Check sheet for the modelled part. Datum: model origin and axes. Units: mm. Face numbers are marked on the shaded views. Round coordinates to 2 decimals unless told otherwise and drop trailing zeros. Loops run counter-clockwise (first coordinate to the right, second up) from the corner with the lowest first, then second, coordinate; pieces in that order, holes last. Notation, with made-up numbers: (40.25, 44) -> (77.25, 44) arc R24 cw to (77.25, 72) -> close; hole circle Ø10 at (85.25, 88.5). An arc over 180 degrees is marked (long way). One line per item, written item: value. Start each with the question number.
1. Release check for a two-part mould opening along Z. For the marked faces 1, 2 and 3 record: +Z half, -Z half, draft (parallel to the pull), parting line (faces both ways), or undercut.
2. Cross-section at A-A on z = 0. Record the cut outline in (x, y), then the cut area to 3 significant figures.
3. Cross-section at C-C on x = 3.8. Record the cut outline in (y, z).
4. Cross-section at D-D on z = -3.75. Record the cut outline in (x, y), then the cut area to 3 significant figures.
5. Material ranges on L1, parallel to Y at x = 4.75, z = 0; L2, parallel to X at y = 16.5, z = -2.25; L3, parallel to Y at x = 3.8, z = 1, recorded low to high.
6. Go/stop test with flat-tipped pins: pin 1 (1.5 mm diameter, centred on x = 4, y = -15.5, fed in from +Z); pin 2 (1 mm diameter, centred on y = 7.5, z = -2, fed in from +X); pin 3 (1.5 mm diameter, centred on x = 1, z = 2, fed in from +Y); pin 4 (2 mm diameter, centred on x = 4.5, z = 1.5, fed in from +Y). Record where each tip stops, or that it passes through.
7. Cross-section at B-B on y = 0. Record the cut outline in (x, z).
from build123d import *

# Parameters (mm, degrees)
SKETCH1_R           = 4.318
BOSS_EXTRUDE1_DEPTH = 5.842
BOSS_EXTRUDE2_DEPTH = 2.6162
SKETCH3_R           = 2.7305
CUT_EXTRUDE1_DEPTH  = 3.2258


with BuildPart() as part:
    # Sketch1 → Boss-Extrude1 (new body)
    with BuildSketch(Plane(origin=(0, 0, 0), x_dir=(0, 0, -1), z_dir=(1, 0, 0))):
        Circle(SKETCH1_R)
    extrude(amount=BOSS_EXTRUDE1_DEPTH)

    # Sketch2 → Boss-Extrude2 (add)
    with BuildSketch(Plane.ZY):
        with BuildLine():
            Line((-2.54, 17.140843061), (-4.226068598, 0.886266441))
            ThreePointArc((-4.226068598, 0.886266441), (0, 4.318), (4.226068598, 0.886266441))
            Line((4.226068598, 0.886266441), (2.54, 17.140843061))
            ThreePointArc((2.54, 17.140843061), (0, 19.431), (-2.54, 17.140843061))
        make_face()
    boss_extrude2 = extrude(amount=-BOSS_EXTRUDE2_DEPTH)

    # Mirror1: Boss-Extrude2 across plane
    add(boss_extrude2.mirror(Plane.ZX))

    # Sketch3 → Cut-Extrude1 (cut)
    with BuildSketch(Plane(origin=(5.842, 0, 0), x_dir=(0, 0, -1), z_dir=(1, 0, 0))):
        Circle(SKETCH3_R)
    extrude(amount=-CUT_EXTRUDE1_DEPTH, mode=Mode.SUBTRACT)


solid = part.part
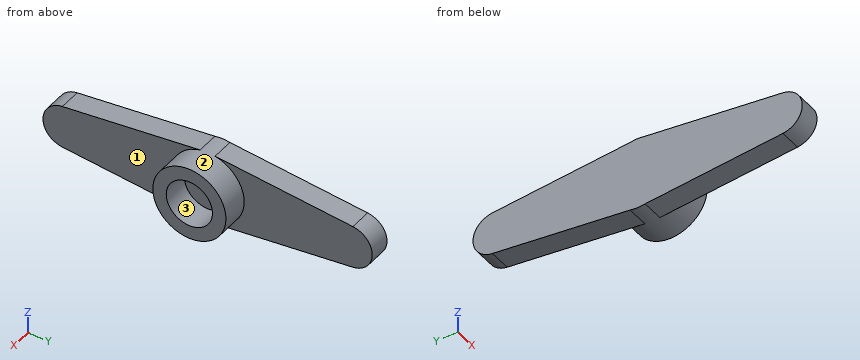
Taken from the geometry:
1. face 1: draft
1. face 2: parting line
1. face 3: undercut
2. outline: (0, -19.43) -> (2.62, -19.43) -> (2.62, -4.32) -> (5.84, -4.32) -> (5.84, -2.73) -> (2.62, -2.73) -> (2.62, 2.73) -> (5.84, 2.73) -> (5.84, 4.32) -> (2.62, 4.32) -> (2.62, 19.43) -> (0, 19.43) -> close
2. area: 112 mm2
3. outline: circle Ø8.64 at (0, 0); hole circle Ø5.46 at (0, 0)
4. outline: (0, -5.48) -> (2.62, -5.48) -> (2.62, -2.14) -> (5.84, -2.14) -> (5.84, 2.14) -> (2.62, 2.14) -> (2.62, 5.48) -> (0, 5.48) -> close
4. area: 42.5 mm2
5. L1: y = -4.32 to -2.73, 2.73 to 4.32
5. L2: x = 0 to 2.62
5. L3: y = -4.2 to -2.54, 2.54 to 4.2
6. pin 1: passes through
6. pin 2: stops at x = 2.62
6. pin 3: stops at y = 19.1
6. pin 4: stops at y = 4.29
7. outline: (0, -4.32) -> (5.84, -4.32) -> (5.84, -2.73) -> (2.62, -2.73) -> (2.62, 2.73) -> (5.84, 2.73) -> (5.84, 4.32) -> (0, 4.32) -> close
